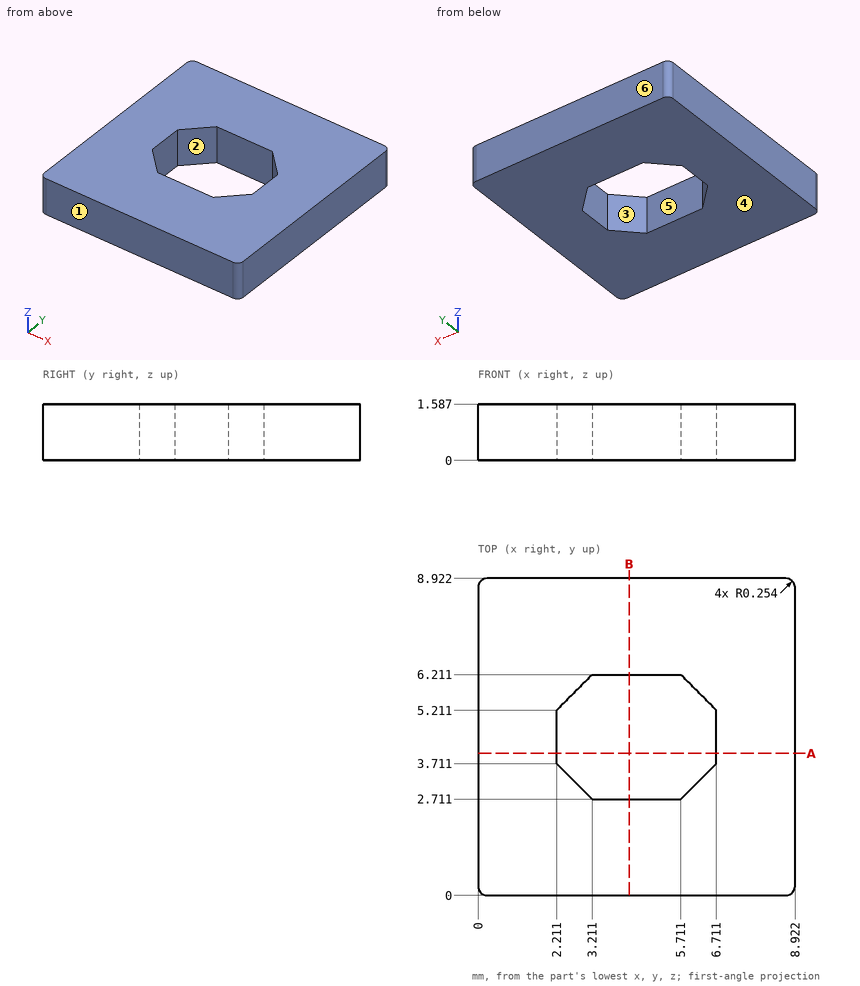
Source: three-view drawing plus pictorial views. Frame: mm from the lowest corner of the part. A direction names the side the tool comes from. Give positions to 0.01 mm unless a question says otherwise; leave off trailing zeros. Write each loop counter-clockwise with the first axis right and the second up, starting at its lowest first coordinate (ties: lowest second). Pieces come first, ordered by that corner, then holes. Notation, with made-up numbers: M 48.25,-14.75 L 87.25,-14.75 A27 cw 87.25,23.25 Z; hole C 56,59 d1. An arc over 180 degrees is marked long. Use one line per item in the form item = value.
1. Cut plane A-A on y = 4. Return loops of the section in (x, z).
Outcome:
outline = M 0,0 L 2.21,0 L 2.21,1.59 L 0,1.59 Z; M 6.71,0 L 8.92,0 L 8.92,1.59 L 6.71,1.59 Z
2. Ray query, L1, parallel to Y at x = 3.5, z = 0.9; L2, parallel to X at y = 4.25, z = 0.65; L3, parallel to X at y = 5.5, z = 0.15 (1 decimal). Return the intervals inside material, ascending.
Outcome:
L1 = 0 to 2.71, 6.21 to 8.92
L2 = 0 to 2.21, 6.71 to 8.92
L3 = 0 to 2.5, 6.4 to 8.9
3. Cut plane B-B on x = 4.25. Return loops of the section in (y, z).
Outcome:
outline = M 0,0 L 2.71,0 L 2.71,1.59 L 0,1.59 Z; M 6.21,0 L 8.92,0 L 8.92,1.59 L 6.21,1.59 Z
4. Reachability of the marked faces 1 and 2 from +Z, -Z, +X, -X, +Y, -Y: full face, straight path, thin tool, end or side. Return the list, or none.
Outcome:
face_1 = +Z, -Z, +X, -X, -Y
face_2 = +Z, -Z
5. Mould query, pull axis Y, two halves, no side actions, for the marked faces 3, 4, 5 and 6. Classes: released by +Y, released by -Y, zero draft, split by the parting line, or undercut.
Outcome:
face_3 = undercut
face_4 = zero draft
face_5 = undercut
face_6 = released by +Y
